```python
from build123d import *

# Parameters (mm, degrees)
SKETCH_1_W                        = 508
SKETCH_1_H                        = 281.5
SKETCH_1_R                        = 3
SKETCH_1_R_2                      = 30
SKETCH_1_W_2                      = 94
SKETCH_1_H_2                      = 46
SM_BASE_FLANGE_1_DEPTH            = 1
SM_EDGE_FLANGE_1_STRIP_W          = 5
SM_EDGE_FLANGE_1_STRIP_H          = 1
SM_EDGE_FLANGE_1_STRIP_CUT_DEPTH  = 408
SM_EDGE_FLANGE_1_RELIEF_W         = 6
SM_EDGE_FLANGE_1_RELIEF_H         = 1
SM_EDGE_FLANGE_1_RELIEF_CUT_DEPTH = 1
SM_EDGE_FLANGE_1_DEPTH            = 408
SM_EDGE_FLANGE_2_STRIP_W          = 5
SM_EDGE_FLANGE_2_STRIP_H          = 1
SM_EDGE_FLANGE_2_STRIP_CUT_DEPTH  = 408
SM_EDGE_FLANGE_2_RELIEF_W         = 6
SM_EDGE_FLANGE_2_RELIEF_H         = 1
SM_EDGE_FLANGE_2_RELIEF_CUT_DEPTH = 1
SM_EDGE_FLANGE_2_DEPTH            = 408
SM_EDGE_FLANGE_3_STRIP_W          = 5
SM_EDGE_FLANGE_3_STRIP_H          = 1
SM_EDGE_FLANGE_3_STRIP_CUT_DEPTH  = 181.5
SM_EDGE_FLANGE_3_RELIEF_W         = 6
SM_EDGE_FLANGE_3_RELIEF_H         = 1
SM_EDGE_FLANGE_3_RELIEF_CUT_DEPTH = 1
SM_EDGE_FLANGE_3_DEPTH            = 181.5
SM_EDGE_FLANGE_4_STRIP_W          = 5
SM_EDGE_FLANGE_4_STRIP_H          = 1
SM_EDGE_FLANGE_4_STRIP_CUT_DEPTH  = 181.5
SM_EDGE_FLANGE_4_RELIEF_W         = 6
SM_EDGE_FLANGE_4_RELIEF_H         = 1
SM_EDGE_FLANGE_4_RELIEF_CUT_DEPTH = 1
SM_EDGE_FLANGE_4_DEPTH            = 181.5
SKETCH_18_R                       = 4
CUT_EXTRUDE_1_DEPTH               = 379.889495764
SKETCH_19_W                       = 92
SKETCH_19_H                       = 18.5
SKETCH_19_W_2                     = 61.5
CUT_EXTRUDE_2_DEPTH               = 379.889495764


# Sheet-metal steps are written as plain solids
with BuildPart() as part:
    # Sketch 1 → 基体-法兰1 (new body)
    with BuildSketch(Plane.XY):
        Rectangle(SKETCH_1_W, SKETCH_1_H)
        with Locations((-244, 130.75)):
            Circle(SKETCH_1_R, mode=Mode.SUBTRACT)
        with Locations((-244, -130.75)):
            Circle(SKETCH_1_R, mode=Mode.SUBTRACT)
        with Locations((244, 130.75)):
            Circle(SKETCH_1_R, mode=Mode.SUBTRACT)
        with Locations((244, -130.75)):
            Circle(SKETCH_1_R, mode=Mode.SUBTRACT)
        with Locations((174, -60.75)):
            Circle(SKETCH_1_R_2, mode=Mode.SUBTRACT)
        with Locations((95.5, 99.75)):
            Rectangle(SKETCH_1_W_2, SKETCH_1_H_2, mode=Mode.SUBTRACT)
    extrude(amount=-SM_BASE_FLANGE_1_DEPTH)

    # 边线-法兰1 strip (across the edge) → 边线-法兰1 strip cut (cut)
    with BuildSketch(Plane(origin=(204, 140.75, 0), x_dir=(0, -1, 0), z_dir=(-1, 0, 0))):
        with Locations((-1, -0.5)):
            Rectangle(SM_EDGE_FLANGE_1_STRIP_W, SM_EDGE_FLANGE_1_STRIP_H)
    extrude(amount=SM_EDGE_FLANGE_1_STRIP_CUT_DEPTH, mode=Mode.SUBTRACT)

    # 边线-法兰1 relief (on the sheet) → 边线-法兰1 relief cut (cut)
    with BuildSketch(Plane(origin=(204, 139.25, 0), x_dir=(0, -1, 0), z_dir=(0, 0, 1))):
        with Locations((-2, 0.5)):
            Rectangle(SM_EDGE_FLANGE_1_RELIEF_W, SM_EDGE_FLANGE_1_RELIEF_H)
        with Locations((-2, -408.5)):
            Rectangle(SM_EDGE_FLANGE_1_RELIEF_W, SM_EDGE_FLANGE_1_RELIEF_H)
    extrude(amount=-SM_EDGE_FLANGE_1_RELIEF_CUT_DEPTH, mode=Mode.SUBTRACT)

    # 边线-法兰1 section (across the edge) → 边线-法兰1 (add)
    with BuildSketch(Plane(origin=(204, 140.75, 0), x_dir=(0, -1, 0), z_dir=(-1, 0, 0))):
        with BuildLine():
            Line((0, 0.5), (0, 19))
            Line((0, 19), (1, 19))
            Line((1, 19), (1, 0.5))
            ThreePointArc((1, 0.5), (1.146446609, 0.146446609), (1.5, 0))
            Line((1.5, 0), (1.5, -1))
            ThreePointArc((1.5, -1), (0.439339828, -0.560660172), (0, 0.5))
        make_face()
    extrude(amount=SM_EDGE_FLANGE_1_DEPTH)

    # 边线-法兰2 strip (across the edge) → 边线-法兰2 strip cut (cut)
    with BuildSketch(Plane(origin=(-204, -140.75, 0), x_dir=(0, 1, 0), z_dir=(1, 0, 0))):
        with Locations((-1, -0.5)):
            Rectangle(SM_EDGE_FLANGE_2_STRIP_W, SM_EDGE_FLANGE_2_STRIP_H)
    extrude(amount=SM_EDGE_FLANGE_2_STRIP_CUT_DEPTH, mode=Mode.SUBTRACT)

    # 边线-法兰2 relief (on the sheet) → 边线-法兰2 relief cut (cut)
    with BuildSketch(Plane(origin=(-204, -139.25, 0), x_dir=(0, 1, 0), z_dir=(0, 0, 1))):
        with Locations((-2, 0.5)):
            Rectangle(SM_EDGE_FLANGE_2_RELIEF_W, SM_EDGE_FLANGE_2_RELIEF_H)
        with Locations((-2, -408.5)):
            Rectangle(SM_EDGE_FLANGE_2_RELIEF_W, SM_EDGE_FLANGE_2_RELIEF_H)
    extrude(amount=-SM_EDGE_FLANGE_2_RELIEF_CUT_DEPTH, mode=Mode.SUBTRACT)

    # 边线-法兰2 section (across the edge) → 边线-法兰2 (add)
    with BuildSketch(Plane(origin=(-204, -140.75, 0), x_dir=(0, 1, 0), z_dir=(1, 0, 0))):
        with BuildLine():
            Line((0, 0.5), (0, 19))
            Line((0, 19), (1, 19))
            Line((1, 19), (1, 0.5))
            ThreePointArc((1, 0.5), (1.146446609, 0.146446609), (1.5, 0))
            Line((1.5, 0), (1.5, -1))
            ThreePointArc((1.5, -1), (0.439339828, -0.560660172), (0, 0.5))
        make_face()
    extrude(amount=SM_EDGE_FLANGE_2_DEPTH)

    # 边线-法兰3 strip (across the edge) → 边线-法兰3 strip cut (cut)
    with BuildSketch(Plane(origin=(254, -90.75, 0), x_dir=(-1, 0, 0), z_dir=(0, 1, 0))):
        with Locations((-1, -0.5)):
            Rectangle(SM_EDGE_FLANGE_3_STRIP_W, SM_EDGE_FLANGE_3_STRIP_H)
    extrude(amount=SM_EDGE_FLANGE_3_STRIP_CUT_DEPTH, mode=Mode.SUBTRACT)

    # 边线-法兰3 relief (on the sheet) → 边线-法兰3 relief cut (cut)
    with BuildSketch(Plane(origin=(252.5, -90.75, 0), x_dir=(-1, 0, 0), z_dir=(0, 0, 1))):
        with Locations((-2, 0.5)):
            Rectangle(SM_EDGE_FLANGE_3_RELIEF_W, SM_EDGE_FLANGE_3_RELIEF_H)
        with Locations((-2, -182)):
            Rectangle(SM_EDGE_FLANGE_3_RELIEF_W, SM_EDGE_FLANGE_3_RELIEF_H)
    extrude(amount=-SM_EDGE_FLANGE_3_RELIEF_CUT_DEPTH, mode=Mode.SUBTRACT)

    # 边线-法兰3 section (across the edge) → 边线-法兰3 (add)
    with BuildSketch(Plane(origin=(254, -90.75, 0), x_dir=(-1, 0, 0), z_dir=(0, 1, 0))):
        with BuildLine():
            Line((0, 0.5), (0, 19))
            Line((0, 19), (1, 19))
            Line((1, 19), (1, 0.5))
            ThreePointArc((1, 0.5), (1.146446609, 0.146446609), (1.5, 0))
            Line((1.5, 0), (1.5, -1))
            ThreePointArc((1.5, -1), (0.439339828, -0.560660172), (0, 0.5))
        make_face()
    extrude(amount=SM_EDGE_FLANGE_3_DEPTH)

    # 边线-法兰4 strip (across the edge) → 边线-法兰4 strip cut (cut)
    with BuildSketch(Plane(origin=(-254, 90.75, 0), x_dir=(1, 0, 0), z_dir=(0, -1, 0))):
        with Locations((-1, -0.5)):
            Rectangle(SM_EDGE_FLANGE_4_STRIP_W, SM_EDGE_FLANGE_4_STRIP_H)
    extrude(amount=SM_EDGE_FLANGE_4_STRIP_CUT_DEPTH, mode=Mode.SUBTRACT)

    # 边线-法兰4 relief (on the sheet) → 边线-法兰4 relief cut (cut)
    with BuildSketch(Plane(origin=(-252.5, 90.75, 0), x_dir=(1, 0, 0), z_dir=(0, 0, 1))):
        with Locations((-2, 0.5)):
            Rectangle(SM_EDGE_FLANGE_4_RELIEF_W, SM_EDGE_FLANGE_4_RELIEF_H)
        with Locations((-2, -182)):
            Rectangle(SM_EDGE_FLANGE_4_RELIEF_W, SM_EDGE_FLANGE_4_RELIEF_H)
    extrude(amount=-SM_EDGE_FLANGE_4_RELIEF_CUT_DEPTH, mode=Mode.SUBTRACT)

    # 边线-法兰4 section (across the edge) → 边线-法兰4 (add)
    with BuildSketch(Plane(origin=(-254, 90.75, 0), x_dir=(1, 0, 0), z_dir=(0, -1, 0))):
        with BuildLine():
            Line((0, 0.5), (0, 19))
            Line((0, 19), (1, 19))
            Line((1, 19), (1, 0.5))
            ThreePointArc((1, 0.5), (1.146446609, 0.146446609), (1.5, 0))
            Line((1.5, 0), (1.5, -1))
            ThreePointArc((1.5, -1), (0.439339828, -0.560660172), (0, 0.5))
        make_face()
    extrude(amount=SM_EDGE_FLANGE_4_DEPTH)

    # 草图18 → 切除-拉伸1 (cut, through all)
    with BuildSketch(Plane(origin=(0, 139.75, 0), x_dir=(-1, 0, 0), z_dir=(0, -1, 0))):
        with Locations(Location((-134.5, -9, 0), (0, 0, 90))):
            Circle(SKETCH_18_R)
        with Locations(Location((-56.5, -9, 0), (0, 0, 90))):
            Circle(SKETCH_18_R)
    extrude(amount=-CUT_EXTRUDE_1_DEPTH, mode=Mode.SUBTRACT)

    # 草图19 → 切除-拉伸2 (cut, through all)
    with BuildSketch(Plane(origin=(0, -139.75, 0), x_dir=(1, 0, 0), z_dir=(0, 1, 0))):
        with Locations((-22.5, -9.75)):
            Rectangle(SKETCH_19_W, SKETCH_19_H)
        with Locations((131.75, -9.75)):
            Rectangle(SKETCH_19_W_2, SKETCH_19_H)
    extrude(amount=-CUT_EXTRUDE_2_DEPTH, mode=Mode.SUBTRACT)


solid = part.part
```
The model under review builds one solid part; all positions refer to its coordinate system, in mm. A direction names the side the tool comes from. Coordinates: 2 decimals unless noted, no trailing zeros. Write each loop counter-clockwise with the first axis right and the second up, starting at its lowest first coordinate (ties: lowest second). Pieces come first, ordered by that corner, then holes.
1) Machinability: for faces 4 (the face through (-137, -139.75, 10)), 5 (the face through (253, -1, 10)), 6 (the face through (-4, 2, 0)), which of the approach directions +Z, -Z, +X, -X, +Y, -Y give a long, thin tool a straight path to every point of the face, cutting with its end or side? Answer none if there is none.
2) We need section D-D on x = -74.5. State the section outline as (y, z) points.
3) We need section A-A on y = 43. State the section outline as (x, z) points.
4) To check wall thickness, follow probe 1 along X at (y, z) = (140, 9); probe 2 along Y at (x, z) = (-244, -0.4); probe 3 along X at (y, z) = (130.75, -0.3). State the ranges of each line that lie inside material, in increasing order.
5) The part is to be moulded in two halves that separate along Y. For faces 1 (the face through (202.615, -51.739, -0.493)), 2 (the face through (-137, -140.75, 10)), 3 (the face through (-254, 1, 10)), say which applies: pulls with the +Y half, pulls with the -Y half, needs draft (parallel to the pull), parting line crosses it, or undercut.
6) Clearance check with flat-ended pins moving along their axes: pin 1 Ø1.1 at (x, y) = (-21.5, -140) entering from +Z; pin 2 Ø1.1 at (y, z) = (-140, 13.5) entering from +X; pin 3 Ø3.5 at (x, y) = (244, -130.75) entering from -Z; pin 4 Ø0.8 at (y, z) = (91, -0.5) entering from -X. State where each tip first meets the part, or that it passes through.
7) We need section B-B on z = 8.25. Count the separate pieces of the cut face and the enclosed holes in it, then the cut area to 3 significant figures.
8) We need section C-C on y = 115.5. State the section outline as (x, z) points.
Answer list:
1. face 4: +Z, +X, -X
1. face 5: +Z, +Y, -Y
1. face 6: +Z
2. outline: (-140.75, 0.5) arc R1.5 ccw to (-139.25, -1) - (139.25, -1) arc R1.5 ccw to (140.75, 0.5) - (140.75, 19) - (139.75, 19) - (139.75, 0.5) arc R0.5 cw to (139.25, 0) - (-139.25, 0) arc R0.5 cw to (-139.75, 0.5) - (-139.75, 19) - (-140.75, 19) - close
3. outline: (-254, 0.5) arc R1.5 ccw to (-252.5, -1) - (252.5, -1) arc R1.5 ccw to (254, 0.5) - (254, 19) - (253, 19) - (253, 0.5) arc R0.5 cw to (252.5, 0) - (-252.5, 0) arc R0.5 cw to (-253, 0.5) - (-253, 19) - (-254, 19) - close
4. probe 1: x = -204 to 52.5, 60.5 to 130.5, 138.5 to 204
4. probe 2: y = -140.75 to -133.75, -127.75 to 127.75, 133.75 to 140.75
4. probe 3: x = -254 to -247, -241 to 241, 247 to 254
5. face 1: undercut
5. face 2: pulls with the -Y half
5. face 3: needs draft
6. pin 1: stops at z = 0.5
6. pin 2: stops at x = 204
6. pin 3: passes through
6. pin 4: stops at x = -253.83
7. separate pieces: 8
7. enclosed holes: 0
7. area: 1,010 mm2
8. outline: (-254, -1) - (48.5, -1) - (48.5, 0) - (-254, 0) - close; (142.5, -1) - (254, -1) - (254, 0) - (142.5, 0) - close
